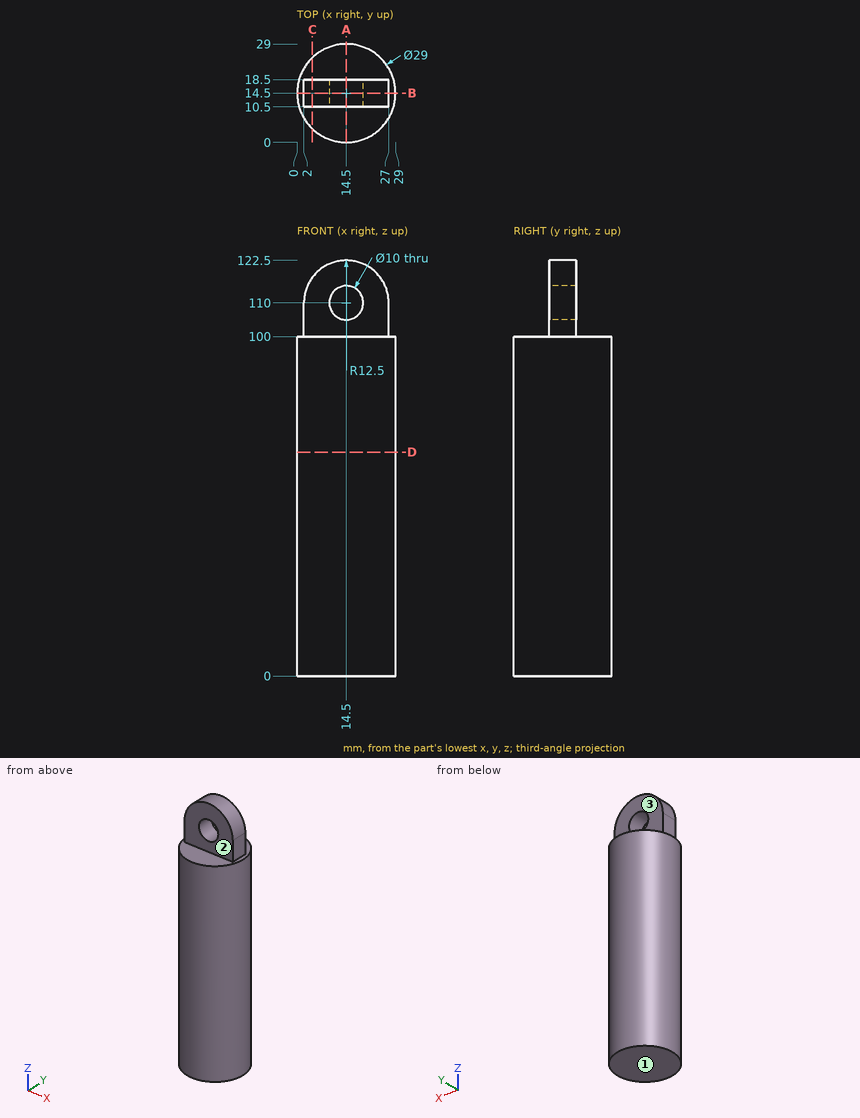
Part print with two shaded views. Sizes in mm from the minimum x, y, z corner. A direction names the side the tool comes from. Coordinates: 2 decimals unless noted, no trailing zeros. Write each loop counter-clockwise with the first axis right and the second up, starting at its lowest first coordinate (ties: lowest second). Pieces come first, ordered by that corner, then holes. Notation, with made-up numbers: (-0.5, 10.5) - (21.5, 10.5) arc R21 cw to (21.5, 44.5) - close; hole circle Ø11 at (41, -14). An arc over 180 degrees is marked (long way). Use a Markdown table: item, result. Add a question column.
Item 1: Band-saw the part on D-D, the plane z = 66. Write the cut outline in (x, y), and give its area (3 significant figures).
Item 2: Band-saw the part on B-B, the plane y = 14.5. Write the cut outline in (x, z), and give its area (3 significant figures).
Item 3: Drop flat-ended pins along their axis: pin 1 (4 mm diameter, centred on x = 11.5, z = 35.5, fed in from -Y); pin 2 (4 mm diameter, centred on y = 16.5, z = 103, fed in from -X); pin 3 (8 mm diameter, centred on x = 25.5, y = 14, fed in from +Z); pin 4 (6 mm diameter, centred on x = 14.5, z = 110, fed in from -Y). Give the stop position or say it passes through.
Item 4: Band-saw the part on A-A, the plane x = 14.5. Write the cut outline in (y, z).
Item 5: Drill centre lines: line 1 along Z through (x, y) = (14.5, 13.75); line 2 along X through (y, z) = (12.75, 107); line 3 along Z through (x, y) = (16.25, 24.25). Where is each one in solid material? Low to high.
Item 6: 3-axis set-ups, long thin cutter, end or side, ignore diameter. For the marked faces 1, 2 and 3: which of +Z, -Z, +X, -X, +Y, -Y reach the whole face in a straight line?
Item 7: Band-saw the part on C-C, the plane x = 4.5. Write the cut outline in (y, z).
A:
| question | item | result |
|---|---|---|
| 1 | outline | circle Ø29 at (14.5, 14.5) |
| 1 | area | 661 mm² |
| 2 | outline | (0, 0) - (29, 0) - (29, 100) - (27, 100) - (27, 110) arc R12.5 ccw to (2, 110) - (2, 100) - (0, 100) - close; hole circle Ø10 at (14.5, 110) |
| 2 | area | 3,320 mm² |
| 3 | pin 1 | stops at y = 0.03 |
| 3 | pin 2 | stops at x = 2 |
| 3 | pin 3 | stops at z = 120.36 |
| 3 | pin 4 | passes through |
| 4 | outline | (0, 0) - (29, 0) - (29, 100) - (18.5, 100) - (18.5, 105) - (10.5, 105) - (10.5, 100) - (0, 100) - close; (10.5, 115) - (18.5, 115) - (18.5, 122.5) - (10.5, 122.5) - close |
| 5 | line 1 | z = 0 to 105, 115 to 122.5 |
| 5 | line 2 | x = 2 to 10.5, 18.5 to 27 |
| 5 | line 3 | z = 0 to 100 |
| 6 | face 1 | -Z, +X, -X, +Y, -Y |
| 6 | face 2 | +Z, +X, -X, -Y |
| 6 | face 3 | +Z, +X, -X, +Y |
| 7 | outline | (4, 0) - (25, 0) - (25, 100) - (18.5, 100) - (18.5, 117.5) - (10.5, 117.5) - (10.5, 100) - (4, 100) - close |
